Could you check a few things on this model? Use its own coordinates, in mm. A direction names the side the tool comes from. Coordinates: 2 decimals unless noted, no trailing zeros. Loops run counter-clockwise (first coordinate to the right, second up) from the corner with the lowest first, then second, coordinate; pieces in that order, holes last. Notation, with made-up numbers: (7, 51) -> (60, 51) arc R19 ccw to (60, 74) -> close; hole circle Ø11 at (-3, 37.5). An arc over 180 degrees is marked (long way). One line per question, with ' | ' between items.
Autodesk Inventor part; units mm, degrees
ref_plane "YZ Plane" through (0, 0, 0) normal (1, 0, 0) x (0, 1, 0)
ref_plane "XZ Plane" through (0, 0, 0) normal (0, 1, 0) x (-1, 0, 0)
ref_plane "XY Plane" through (0, 0, 0) normal (0, 0, 1) x (1, 0, 0)
sketch "Boceto1" plane through (0, 0, 0) normal (0, 1, 0) x (-1, 0, 0)
  line L0 (88, 0) -> (0, 0)
  line L1 (0, 0) -> (0, 58.5)
  line L2 (0, 58.5) -> (88, 58.5)
  line L3 (88, 58.5) -> (88, 0)
  dimension "d0" = 58.5
  dimension "d1" = 88
extrude "Extrusión1" add sketch "Boceto1" along normal blind 24.5
sketch "Boceto2" plane through (0, 24.5, 0) normal (0, 1, 0) x (1, 0, 0)
  line L0 (0, 0) -> (-88, 0)
  line L1 (-88, 0) -> (-88, -58.5)
  line L2 (-88, -58.5) -> (0, -58.5)
  line L3 (0, -58.5) -> (0, 0)
  line L4 (-36, -58.5) -> (0, -58.5)
  line L5 (-36.5, -58.5) -> (-38.5, -58.5)
  line L6 (-39, -58) -> (-39, -40)
  line L7 (-38.5, -39.5) -> (-36.5, -39.5)
  line L8 (-36, -40) -> (-36, -58)
  line L9 (0, 0) -> (-22.5, 0)
  line L10 (-22.5, 0) -> (-82.5, 0)
  line L11 (-82.5, 0) -> (-82.5, -8)
  line L12 (-80.5, -10) -> (-24.5, -10)
  line L13 (-22.5, -8) -> (-22.5, 0)
  arc A0 (-24.5, -10) -> (-22.5, -8) centre (-24.5, -8) ccw
  arc A1 (-82.5, -8) -> (-80.5, -10) centre (-80.5, -8) ccw
  arc A2 (-38.5, -39.5) -> (-39, -40) centre (-38.5, -40) ccw
  arc A3 (-36, -40) -> (-36.5, -39.5) centre (-36.5, -40) ccw
  arc A4 (-36.5, -58.5) -> (-36, -58) centre (-36.5, -58) ccw
  arc A5 (-39, -58) -> (-38.5, -58.5) centre (-38.5, -58) ccw
  line L14 (0, 0) -> (-86, 0)
  line L15 (-86, 0) -> (-86, -58.5)
  line L16 (-86, -58.5) -> (0, -58.5)
  line L17 (0, -58.5) -> (0, 0)
  line L18 (-38.6961, -58.4599) -> (-36.3039, -58.4599)
  point P0 (-39, -39.5)
  point P1 (-36, -39.5)
  dimension "d4" = 36
  dimension "d5" = 19
  dimension "d6" = 3
  dimension "d7" = 22.5
  dimension "d8" = 2
  dimension "d9" = 0.5
  dimension "d10" = 56
  dimension "d11" = 88
  dimension "d12" = 58.5
  dimension "d13" = 86
  dimension "d14" = 10
  dimension "d15" = 2.3923
extrude "Extrusión2" cut sketch "Boceto2" against normal blind 11 contours L13 A0 L12 A1 L11 L0 | L15 L2 L1 L0 | L18 A5 L6 A2 L7 A3 L8 A4
sketch "Boceto3" plane through (0, 24.5, 0) normal (0, 1, 0) x (1, 0, 0)
  line L0 (-86, 0) -> (-86, -58.5)
  line L1 (-86, -58.5) -> (0, -58.5)
  line L2 (0, -58.5) -> (0, 0)
  line L3 (0, 0) -> (-22.5, 0)
  line L4 (-22.5, 0) -> (-22.5, -8)
  arc A0 (-24.5, -10) -> (-22.5, -8) centre (-24.5, -8) ccw
  line L5 (-24.5, -10) -> (-80.5, -10)
  arc A1 (-82.5, -8) -> (-80.5, -10) centre (-80.5, -8) ccw
  line L6 (-82.5, -8) -> (-82.5, 0)
  line L7 (-82.5, 0) -> (-86, 0)
  line L8 (-39, -58) -> (-39, -40)
  arc A2 (-38.5, -39.5) -> (-39, -40) centre (-38.5, -40) ccw
  line L9 (-38.5, -39.5) -> (-36.5, -39.5)
  arc A3 (-36, -40) -> (-36.5, -39.5) centre (-36.5, -40) ccw
  line L10 (-36, -40) -> (-36, -58)
  arc A4 (-36.3039, -58.4599) -> (-36, -58) centre (-36.5, -58) ccw
  line L11 (-36.3039, -58.4599) -> (-38.6961, -58.4599)
  arc A5 (-39, -58) -> (-38.6961, -58.4599) centre (-38.5, -58) ccw
sketch "Boceto4" plane through (0, 13.5, 0) normal (0, 1, 0) x (1, 0, 0)
  line L0 (-88, -58.5) -> (-88, 0)
  line L1 (-86, -58.5) -> (-88, -58.5)
  line L2 (-88, 0) -> (-86, 0)
  line L3 (-86, 0) -> (-86, -58.5)
  line L4 (-86, -58.5) -> (-88, -58.5)
  line L5 (-88, -58.5) -> (-88, 0)
  point P0 (0, 0)
extrude "Extrusión3" cut sketch "Boceto4" against normal blind 50
chamfer "Chaflán1" distance 2 angle 45 1 edges at (0, 12.25, 58.5)
chamfer "Chaflán2" distance 2 angle 45 1 edges at (0, 12.25, 0)
chamfer "Chaflán3" distance 2 angle 45 1 edges at (-86, 12.25, 58.5)
chamfer "Chaflán4" distance 2 angle 45 1 edges at (-86, 12.25, 0)
properties part number "Rasp" material "Policarbonato, ahumado"
1) I need wall thicknesses on line 1 along X through (y, z) = (15, 55); line 2 along X through (y, z) = (19, 6); line 3 along Z through (x, y) = (-42.5, 17). Which ranges of each line are inside material? Lowest first, please. Write a range as from..to.
Data:
line 1: -86..-39, -36..0 | line 2: -86..-82.5, -22.5..0 | line 3: 10..58.5
2) If we section it at B-B on y = 19.5: Please give me the cut outline in (x, z), and give its area (3 significant figures).
Data:
outline: (-86, 2) -> (-84, 0) -> (-82.5, 0) -> (-82.5, 8) arc R2 cw to (-80.5, 10) -> (-24.5, 10) arc R2 cw to (-22.5, 8) -> (-22.5, 0) -> (-2, 0) -> (0, 2) -> (0, 56.5) -> (-2, 58.5) -> (-84, 58.5) -> (-86, 56.5) -> close; hole (-39, 40) arc R0.5 ccw to (-38.5, 39.5) -> (-36.5, 39.5) arc R0.5 ccw to (-36, 40) -> (-36, 58) arc R0.5 ccw to (-36.3, 58.46) -> (-38.7, 58.46) arc R0.5 ccw to (-39, 58) -> close | area: 4,370 mm²
3) We'd pull the mould along X, two halves only. Please class faces 4 (the face through (-38, 13.5, 49)), 5 (the face through (-42, 12, 58.5)), 6 (the face through (0, 12, 29)), 7 (the face through (-36, 19, 49)): pulls with the +X half, pulls with the -X half, needs draft (parallel to the pull), parting line crosses it, or undercut.
Data:
face 4: undercut | face 5: needs draft | face 6: pulls with the +X half | face 7: undercut
4) I'm going to push flat-ended pins straight in: pin 1 Ø10 at (x, y) = (-11, 8) entering from -Z; pin 2 Ø5 at (x, z) = (-64.5, 7) entering from +Y; pin 3 Ø1.5 at (x, y) = (-50, 17.5) entering from -Z. Where does each tip first touch, or does it pass through?
Data:
pin 1: z = 0 | pin 2: y = 13.5 | pin 3: z = 10
5) If we section it at C-C on x = -52.5: Please give me the cut outline in (y, z), and give its area (3 significant figures).
Data:
outline: (0, 0) -> (13.5, 0) -> (13.5, 10) -> (24.5, 10) -> (24.5, 58.5) -> (0, 58.5) -> close | area: 1,320 mm²
6) If we section it at A-A on z = 48.5: Please give me the cut outline in (x, y).
Data:
outline: (-86, 0) -> (0, 0) -> (0, 24.5) -> (-36, 24.5) -> (-36, 13.5) -> (-39, 13.5) -> (-39, 24.5) -> (-86, 24.5) -> close
7) On a 3-axis mill with a long thin cutter (end or side, diameter ignored), from which of +Z, -Z, +X, -X, +Y, -Y can I reach the whole of each face in a straight line? I mean faces 1 (the face through (-22.5, 19, 4)), 2 (the face through (-39, 19, 49)), 3 (the face through (-42, 24.5, 30)). Say none if no direction works.
Data:
face 1: -Z, +Y | face 2: +Y | face 3: +Z, -Z, +X, -X, +Y
